```python
from build123d import *

# Parameters (mm, degrees)
F0_W     = 20
F0_H     = 100
F1_DEPTH = 20
F2_R     = 6
F3_DEPTH = 2.5
F4_R     = 4
F5_DEPTH = 10
F7_DEPTH = 25


with BuildPart() as f1:
    # F0 (on Top) → F1 (new body)
    with BuildSketch(Plane.XY):
        Rectangle(F0_W, F0_H)
    extrude(amount=F1_DEPTH)

    # F2 (on face) → F3 (cut)
    with BuildSketch(Plane.YZ.offset(10)):
        with Locations((0, 10)):
            Circle(F2_R)
    extrude(amount=-F3_DEPTH, mode=Mode.SUBTRACT)

    # F4 (on face) → F5 (cut)
    with BuildSketch(Plane.YZ.offset(10)):
        with Locations((22.5, 10)):
            Circle(F4_R)
        with Locations((-22.5, 10)):
            Circle(F4_R)
    extrude(amount=-F5_DEPTH, mode=Mode.SUBTRACT)

    # F6 (on face) → F7 (cut)
    with BuildSketch(Plane.YZ.offset(10)):
        with BuildLine():
            ThreePointArc((-37.9, 10), (-40, 12.1), (-42.1, 10))
            Line((-42.1, 10), (-37.9, 10))
        make_face()
        with BuildLine():
            Line((-37.9, 10), (-42.1, 10))
            ThreePointArc((-42.1, 10), (-40, 7.9), (-37.9, 10))
        make_face()
        with BuildLine():
            ThreePointArc((37.9, 10), (40, 7.9), (42.1, 10))
            Line((42.1, 10), (37.9, 10))
        make_face()
        with BuildLine():
            Line((37.9, 10), (42.1, 10))
            ThreePointArc((42.1, 10), (40, 12.1), (37.9, 10))
        make_face()
    extrude(amount=-F7_DEPTH, mode=Mode.SUBTRACT)


solid = f1.part
```
Work out the finished part from the listing and answer in its coordinate system (mm). A direction names the side the tool comes from. Give positions to 0.01 mm unless a question says otherwise; leave off trailing zeros. Order: outer loops, then holes, each group sorted by start corner. A loop starts at its lowest first (then second) coordinate and runs counter-clockwise, first axis right, second up. Notation, with made-up numbers: (49, -14.5) - (104, -14.5) arc R5 cw to (104, -6.5) - close; hole circle Ø11 at (57, 1.25). An arc over 180 degrees is marked (long way). One line per item, written item: value. Start each with the question number.
1. Section B-B, the plane x = 2.25 is taken. Write down the section's boundary in (y, z), then the cut area to 3 significant figures.
2. Which of the six approach directions +Z, -Z, +X, -X, +Y, -Y give full straight-line access (tool end or side, diameter ignored) to faces 1 (the face through (0, 50, 10)), 2 (the face through (0, -23, 10))?
3. Section A-A, the plane y = 40 is taken. Write down the section's boundary in (x, z).
4. Each of these flat-tipped pins is pushed along its axis until it touches: pin 1 Ø2.5 at (y, z) = (21.5, 11) entering from +X; pin 2 Ø3.5 at (y, z) = (-0.5, 8) entering from +X. Where does it stop, or does it pass through?
5. For a pull along Y with two mould halves and no side action, classify faces 3 (the face through (0, -50, 10)), 4 (the face through (10, -1, 3)), 5 (the face through (5.07, 18.504, 10.176)) as released by +Y, released by -Y, zero draft, split by the parting line, or undercut.
6. Consider line 1 (Y direction, x = 7.25, z = 10.75); line 2 (Z direction, x = 9.1, y = 0); line 3 (Y direction, x = -5.5, z = 10.75). Determine where each line is inside the solid, lowest interval first.
7. Section C-C, the plane z = 10 is taken. Write down the section's boundary in (x, y), then the cut area to 3 significant figures.
8. Section D-D, the plane y = -22.5 is taken. Write down the section's boundary in (x, z), then the cut area to 3 significant figures.
Filled sheet:
1. outline: (-50, 0) - (50, 0) - (50, 20) - (-50, 20) - close; hole circle Ø4.2 at (-40, 10); hole circle Ø8 at (-22.5, 10); hole circle Ø8 at (22.5, 10); hole circle Ø4.2 at (40, 10)
1. area: 1,870 mm²
2. face 1: +Z, -Z, +X, -X, +Y
2. face 2: +X
3. outline: (-10, 0) - (10, 0) - (10, 7.9) - (-10, 7.9) - close; (-10, 12.1) - (10, 12.1) - (10, 20) - (-10, 20) - close
4. pin 1: x = 0
4. pin 2: x = 7.5
5. face 3: released by -Y
5. face 4: zero draft
5. face 5: undercut
6. line 1: -50 to -41.96, -38.04 to -26.43, -18.57 to 18.57, 26.43 to 38.04, 41.96 to 50
6. line 2: 0 to 4, 16 to 20
6. line 3: -50 to -41.96, -38.04 to 38.04, 41.96 to 50
7. outline: (-10, -50) - (10, -50) - (10, -42.1) - (-10, -42.1) - close; (-10, -37.9) - (10, -37.9) - (10, -26.5) - (0, -26.5) - (0, -18.5) - (10, -18.5) - (10, -6) - (7.5, -6) - (7.5, 6) - (10, 6) - (10, 18.5) - (0, 18.5) - (0, 26.5) - (10, 26.5) - (10, 37.9) - (-10, 37.9) - close; (-10, 42.1) - (10, 42.1) - (10, 50) - (-10, 50) - close
7. area: 1,640 mm²
8. outline: (-10, 0) - (10, 0) - (10, 6) - (0, 6) - (0, 14) - (10, 14) - (10, 20) - (-10, 20) - close
8. area: 320 mm²
